from build123d import *

# Parameters (mm, degrees)
SKETCH_1_W          = 60
SKETCH_1_H          = 60
EXTRUDE_1_DEPTH     = 10
SKETCH_2_W          = 60
SKETCH_2_H          = 10
SKETCH_2_R          = 3
CUT_EXTRUDE_1_DEPTH = 10
SKETCH_3_R          = 5
CUT_EXTRUDE_2_DEPTH = 44.588989435


with BuildPart() as part:
    # 草图1 → 凸台-拉伸1 (new body)
    with BuildSketch(Plane.XY):
        Rectangle(SKETCH_1_W, SKETCH_1_H)
    extrude(amount=EXTRUDE_1_DEPTH)

    # 草图2 → 切除-拉伸1 (cut)
    with BuildSketch(Plane(origin=(0, 30, 0), x_dir=(1, 0, 0), z_dir=(0, 1, 0))):
        with Locations((0, -5)):
            Rectangle(SKETCH_2_W, SKETCH_2_H)
        with Locations(Location((0, -5, 0), (0, 0, 270))):
            Circle(SKETCH_2_R, mode=Mode.SUBTRACT)
    extrude(amount=-CUT_EXTRUDE_1_DEPTH, mode=Mode.SUBTRACT)

    # 草图3 → 切除-拉伸2 (cut, through all)
    with BuildSketch(Plane.XY.offset(10)):
        with Locations((-20, -20)):
            Circle(SKETCH_3_R)
        with Locations((20, 10)):
            Circle(SKETCH_3_R)
    extrude(amount=-CUT_EXTRUDE_2_DEPTH, mode=Mode.SUBTRACT)


solid = part.part
Could you check a few things on this model? Use its own coordinates, in mm. A direction names the side the tool comes from. Coordinates: 2 decimals unless noted, no trailing zeros. Order: outer loops, then holes, each group sorted by start corner. A loop starts at its lowest first (then second) coordinate and runs counter-clockwise, first axis right, second up.
Q1. Which directions (+Z, -Z, +X, -X, +Y, -Y) give clear straight access to the entire face, cutting with the end or side of a thin tool? Please do faces 4 (the flat face through (0, -5, 10)), 5 (the cylindrical face through (0, 25, 2)).
Q2. Will these pins go through, and if not, where does the flat tip stop? pin 1 (1 mm diameter, centred on x = -5.5, z = 1, fed in from +Y); pin 2 (2 mm diameter, centred on x = -22.5, y = 14.5, fed in from -Z).
Q3. Thinking about a two-plate mould opening in X: for faces 1 (the flat face through (-0.4, 20, 1.6)), 2 (the flat face through (-30, -5, 5)), 3 (the cylindrical face through (-21.08, -24.88, 5.07)), which applies, released by +X, released by -X, zero draft, split by the parting line, or undercut?
Q4. Suppose I cut it at B-B on y = 10. Please give me the cut outline in (x, z).
Q5. Suppose I cut it at C-C on z = 5. Please give me the cut outline in (x, y), and give its area (3 significant figures).
Q6. Suppose I cut it at D-D on x = 0. Please give me the cut outline in (y, z).
Q7. Suppose I cut it at A-A on x = 20. Please give me the cut outline in (y, z).
Q8. Please list where these lines run through material, in increasing order: L1, parallel to Y at x = -20, z = 2; L2, parallel to Y at x = 20, z = 7.25; L3, parallel to Y at x = 25.5, z = 3.25.
Answer:
1. face 4: +Z, +X, -X, +Y, -Y
1. face 5: +Y
2. pin 1: stops at y = 20
2. pin 2: stops at z = 0
3. face 1: zero draft
3. face 2: released by -X
3. face 3: undercut
4. outline: (-30, 0) - (15, 0) - (15, 10) - (-30, 10) - close; (25, 0) - (30, 0) - (30, 10) - (25, 10) - close
5. outline: (-30, -30) - (30, -30) - (30, 20) - (3, 20) - (3, 30) - (-3, 30) - (-3, 20) - (-30, 20) - close; hole circle Ø10 at (-20, -20); hole circle Ø10 at (20, 10)
5. area: 2,900 mm2
6. outline: (-30, 0) - (20, 0) - (20, 2) - (30, 2) - (30, 8) - (20, 8) - (20, 10) - (-30, 10) - close
7. outline: (-30, 0) - (5, 0) - (5, 10) - (-30, 10) - close; (15, 0) - (20, 0) - (20, 10) - (15, 10) - close
8. L1: y = -30 to -25, -15 to 20
8. L2: y = -30 to 5, 15 to 20
8. L3: y = -30 to 20
